Autodesk Inventor part; units mm, degrees
ref_plane "YZ Plane" through (0, 0, 0) normal (1, 0, 0) x (0, 1, 0)
ref_plane "XZ Plane" through (0, 0, 0) normal (0, 1, 0) x (-1, 0, 0)
ref_plane "XY Plane" through (0, 0, 0) normal (0, 0, 1) x (1, 0, 0)
sketch "Sketch1" plane through (0, 0, 0) normal (0, 0, 1) x (1, 0, 0)
  line L0 (0, 0) -> (254, 0)
  line L1 (254, 0) -> (254, 254)
  line L2 (254, 254) -> (0, 254)
  line L3 (0, 254) -> (0, 0)
  line L4 (25.4, 228.6) -> (228.6, 228.6)
  line L5 (228.6, 228.6) -> (228.6, 25.4)
  line L6 (228.6, 25.4) -> (25.4, 25.4)
  line L7 (25.4, 25.4) -> (25.4, 228.6)
  dimension "d0" = 254
  dimension "d1" = 25.4
extrude "Extrusion1" add sketch "Sketch1" along normal blind 254
sketch "Sketch2" plane through (0, 254, 0) normal (0, 1, 0) x (1, 0, 0)
  line L0 (254, 0) -> (0, 0)
  line L1 (0, 0) -> (0, -254)
  line L2 (254, -254) -> (0, -254)
  line L3 (254, 0) -> (254, -254)
  line L4 (25.4, -228.6) -> (25.4, -25.4)
  line L5 (25.4, -25.4) -> (228.6, -25.4)
  line L6 (228.6, -25.4) -> (228.6, -228.6)
  line L7 (228.6, -228.6) -> (25.4, -228.6)
  dimension "d4" = 25.4
extrude "Extrusion2" cut sketch "Sketch2" against normal blind 254 contours L4 L5 L6 L7
sketch "Sketch3" plane through (254, 0, 0) normal (1, 0, 0) x (0, 0, -1)
  line L0 (0, 0) -> (0, 254)
  line L1 (0, 254) -> (-254, 254)
  line L2 (-254, 0) -> (-254, 254)
  line L3 (0, 0) -> (-254, 0)
  line L4 (0, 0) -> (0, 254)
  line L5 (-25.4, 228.6) -> (-25.4, 25.4)
  line L6 (-25.4, 25.4) -> (-228.6, 25.4)
  line L7 (-228.6, 25.4) -> (-228.6, 228.6)
  line L8 (-228.6, 228.6) -> (-25.4, 228.6)
  dimension "d7" = 25.4
extrude "Extrusion3" cut sketch "Sketch3" against normal blind 254 contours L5 L6 L7 L8
properties part number "CUBE for Game Design_1"
CAD build for the part. Positions are in the model's coordinates, mm. A direction names the side the tool comes from. Round coordinates to 2 decimals unless told otherwise and drop trailing zeros. Loops run counter-clockwise (first coordinate to the right, second up) from the corner with the lowest first, then second, coordinate; pieces in that order, holes last. Notation, with made-up numbers: (-34.5, 88.25) - (-5.5, 88.25) arc R20 ccw to (-5.5, 120.25) - close; hole circle Ø9 at (54, 21.5). An arc over 180 degrees is marked (long way). Put each result on its own line as item: value.
1. Slice it at C-C on x = 17. List the corners of the cut face in (y, z).
Geometry check:
outline: (0, 0) - (254, 0) - (254, 254) - (0, 254) - close; hole (25.4, 25.4) - (228.6, 25.4) - (228.6, 228.6) - (25.4, 228.6) - close
2. Slice it at A-A on y = 213. List the corners of the cut face in (x, z), and give its area (3 significant figures).
Geometry check:
outline: (0, 0) - (25.4, 0) - (25.4, 25.4) - (0, 25.4) - close; (0, 228.6) - (25.4, 228.6) - (25.4, 254) - (0, 254) - close; (228.6, 0) - (254, 0) - (254, 25.4) - (228.6, 25.4) - close; (228.6, 228.6) - (254, 228.6) - (254, 254) - (228.6, 254) - close
area: 2,580 mm²
3. Two-plate mould, pull along Y, no slides. Class faces 1 (the flat face through (228.6, 13, 126)), 2 (the flat face through (25.4, 128, 241)), 3 (the flat face through (238, 0, 125)): released by +Y, released by -Y, zero draft, split by the parting line, or undercut.
Geometry check:
face 1: zero draft
face 2: undercut
face 3: released by -Y
4. 3-axis set-ups, long thin cutter, end or side, ignore diameter. For faces 4 (the flat face through (25.4, 128, 13)), 5 (the flat face through (254, 238, 125)), 6 (the flat face through (242, 254, 125)), 7 (the flat face through (126, 13, 25.4)), 8 (the flat face through (241, 228.6, 128)): which of +Z, -Z, +X, -X, +Y, -Y reach the whole face in a straight line?
Geometry check:
face 4: +Z, -Z
face 5: +Z, -Z, +X, +Y, -Y
face 6: +Z, -Z, +X, -X, +Y
face 7: +Y, -Y
face 8: +X, -X
5. Wall check: line 1 (Y direction, x = 55.5, z = 23.5). Give the ranges that are in metal, low to high.
Geometry check:
line 1: 0 to 25.4, 228.6 to 254
